```python
from build123d import *

# Parameters (mm, degrees)
F0_R     = 9.5
F0_R_2   = 4
F1_DEPTH = 3
F2_SIZE  = 0.5
F3_R     = 8.25
F3_R_2   = 5.5
F4_DEPTH = 0.1
F5_R     = 8.25
F5_R_2   = 5.5
F6_DEPTH = 0.1


with BuildPart() as f1:
    # F0 (on Top) → F1 (new body, symmetric)
    with BuildSketch(Plane.XY):
        Circle(F0_R)
        Circle(F0_R_2, mode=Mode.SUBTRACT)
    extrude(amount=F1_DEPTH, both=True)

    # F2
    f2_edges = [f1.edges().sort_by_distance(p)[0] for p in [
        (-9.5, 0, 3),
        (-4, 0, 3),
        (-9.5, 0, -3),
        (-4, 0, -3),
    ]]
    chamfer(f2_edges, length=F2_SIZE)

    # F3 (on face) → F4 (cut)
    with BuildSketch(Plane(origin=(0, 0, -3), x_dir=(1, 0, 0), z_dir=(0, 0, -1))):
        Circle(F3_R)
        Circle(F3_R_2, mode=Mode.SUBTRACT)
    extrude(amount=-F4_DEPTH, mode=Mode.SUBTRACT)

    # F5 (on face) → F6 (cut)
    with BuildSketch(Plane.XY.offset(3)):
        Circle(F5_R)
        Circle(F5_R_2, mode=Mode.SUBTRACT)
    extrude(amount=-F6_DEPTH, mode=Mode.SUBTRACT)


solid = f1.part
```
Could you check a few things on this model? Use its own coordinates, in mm. A direction names the side the tool comes from. Give positions to 0.01 mm unless a question says otherwise; leave off trailing zeros. Order: outer loops, then holes, each group sorted by start corner. A loop starts at its lowest first (then second) coordinate and runs counter-clockwise, first axis right, second up.
Q1. If I drill on line 1 along Y through (x, z) = (0, -0.3); line 2 along X through (y, z) = (0, -2.95); line 3 along Z through (x, y) = (5.5, -5.5), over which ranges is the centre line in solid material (lowest first)?
Q2. Suppose I cut it at C-C, the plane z = -1.2. Write out the boundary of the cut face in (x, y).
Q3. I'm going to push flat-ended pins straight in: P1, Ø1.5, axis at x = -0.5, z = 0.5, coming from the +Y side; P2, Ø6.5, axis at x = 0, y = 0, coming from the +Z side; P3, Ø2, axis at x = -4.5, z = 0, coming from the -Y side; P4, Ø5, axis at x = -0.5, y = 1.5, coming from the -Z side. Where does each tip first touch, or does it pass through?
Q4. For faces 4 (the flat face through (5.4, 1.7, -2.9)), 5 (the cylindrical face through (-0.867, -3.905, -0.035)), which set-ups out of +Z, -Z, +X, -X, +Y, -Y let a thin tool reach every point of the face, with its end or its side?
Q5. We'd pull the mould along X, two halves only. Please class faces 1 (the flat face through (5.4, -1.7, 2.9)), 2 (the flat face through (-5, 0, 3)), 3 (the cylindrical face through (4.38, -8.43, 0.04)): +X half, -X half, draft (parallel to the pull), parting line (faces both ways), or undercut.
Solution:
1. line 1: y = -9.5 to -4, 4 to 9.5
1. line 2: x = -9.05 to -8.25, -5.5 to -4.45, 4.45 to 5.5, 8.25 to 9.05
1. line 3: z = -2.9 to 2.9
2. outline: circle Ø19 at (0, 0); hole circle Ø8 at (0, 0)
3. P1: stops at y = 9.5
3. P2: passes through
3. P3: stops at y = -8.83
3. P4: stops at z = -2.58
4. face 4: -Z
4. face 5: +Z, -Z
5. face 1: undercut
5. face 2: draft
5. face 3: parting line
